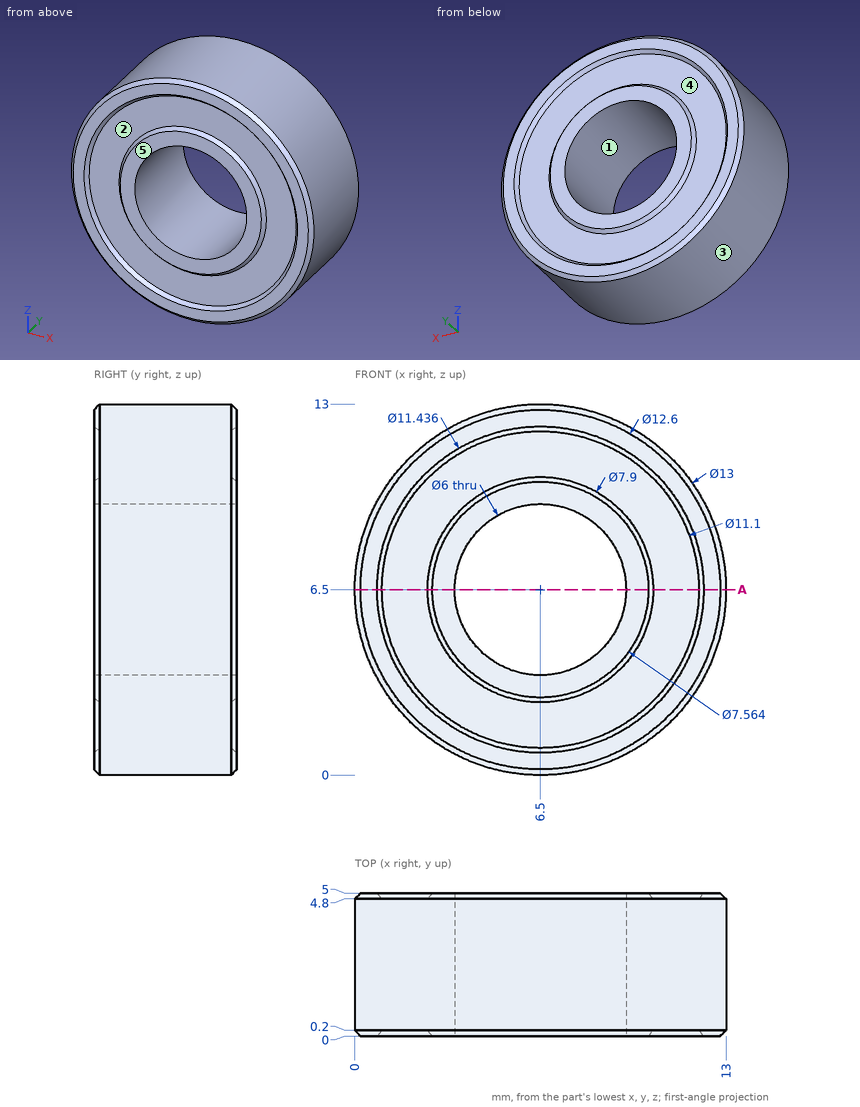
Input: dimensioned drawing with shaded views. Units: mm. Origin: part minimum x, y, z. A direction names the side the tool comes from. Give positions to 0.01 mm unless a question says otherwise; leave off trailing zeros. Loops run counter-clockwise (first coordinate to the right, second up) from the corner with the lowest first, then second, coordinate; pieces in that order, holes last. Notation, with made-up numbers: (-5, -21.5) -> (7, -21.5) arc R19 ccw to (7, -10.5) -> close; hole circle Ø4 at (68.25, 40.5). An arc over 180 degrees is marked (long way). Return JSON: item names as keys, results as strings.
Item 1: Section A-A, the plane z = 6.5. Output: boundary loops of the cut face in (x, y), plus the area to 3 significant figures.
Filled in:
{"outline": "(0, 0.2) -> (0.2, 0) -> (0.78, 0) -> (0.95, 0.2) -> (2.55, 0.2) -> (2.72, 0) -> (3.5, 0) -> (3.5, 5) -> (2.72, 5) -> (2.55, 4.8) -> (0.95, 4.8) -> (0.78, 5) -> (0.2, 5) -> (0, 4.8) -> close; (9.5, 0) -> (10.28, 0) -> (10.45, 0.2) -> (12.05, 0.2) -> (12.22, 0) -> (12.8, 0) -> (13, 0.2) -> (13, 4.8) -> (12.8, 5) -> (12.22, 5) -> (12.05, 4.8) -> (10.45, 4.8) -> (10.28, 5) -> (9.5, 5) -> close", "area": "33.5 mm^2"}
Item 2: Access query for the marked faces 1 and 2. Directions: +Z, -Z, +X, -X, +Y, -Y. A direction counts if a zero-diameter tool reaches every point of the face in a straight line with its end or side. Return the directions, or none.
Filled in:
{"face 1": "+Y, -Y", "face 2": "-Y"}
Item 3: Line query: line 1 (X direction, y = 2.7, z = 6.5); line 2 (X direction, y = 1.5, z = 8.25) (1 decimal); line 3 (Z direction, x = 4, y = 3.65). Output: solid intervals per line, ascending.
Filled in:
{"line 1": "0 to 3.5, 9.5 to 13", "line 2": "0.2 to 4.1, 8.9 to 12.8", "line 3": "0.5 to 4.84, 8.16 to 12.5"}
Item 4: Pin query (flat end, axial travel): P1, Ø1, axis at y = 1.5, z = 4.5, coming from the -X side (1 decimal). Return the tip coordinate at first contact, or that it passes through.
Filled in:
{"P1": "x = 0.2"}
Item 5: Mould query, pull axis Z, two halves, no side actions, for the marked faces 3, 4 and 5. Classes: released by +Z, released by -Z, zero draft, split by the parting line, or undercut.
Filled in:
{"face 3": "split by the parting line", "face 4": "undercut", "face 5": "zero draft"}
